Input: part model. Units: mm. Frame: model coordinates. Face numbers are marked on the shaded views. A direction names the side the tool comes from. Round coordinates to 2 decimals unless told otherwise and drop trailing zeros. Loops run counter-clockwise (first coordinate to the right, second up) from the corner with the lowest first, then second, coordinate; pieces in that order, holes last. Notation, with made-up numbers: (47.5, 75) - (74.5, 75) arc R7 cw to (74.5, 88) - close; hole circle Ø1 at (67, 34.5). An arc over 180 degrees is marked (long way). Use CSV: the item, a comma, the result in double quotes. Start each with the question number.
1. Pull-direction query (X, two-part tool) for the marked faces 3, 4 and 5; classes: +X half, -X half, draft (parallel to the pull), parting line (faces both ways), or undercut.
2. Cut plane C-C (x = -15). Return loops of the section in (y, z), and give its area (3 significant figures).
3. Cut plane A-A (z = 19). Return loops of the section in (x, y).
4. Material intervals for probe 1 along Y at (x, z) = (-14.4, 19); probe 2 along X at (y, z) = (-44.5, 1.75); probe 3 along Y at (x, z) = (-15.5, 21), sorted ascending. Write a range as from..to.
5. Pin query (flat end, axial travel): P1, Ø1.8, axis at y = -24.39, z = 9, coming from the -X side; P2, Ø0.8, axis at x = -15.5, z = 15.5, coming from the -Y side; P3, Ø6.5, axis at y = -38.43, z = 22, coming from the -X side; P4, Ø2.5, axis at y = -24.39, z = 19, coming from the +X side. Return the tip coordinate at first contact, or that it passes through.
6. Access query for the marked faces 1 and 2. Directions: +Z, -Z, +X, -X, +Y, -Y. A direction counts if a zero-diameter tool reaches every point of the face in a straight line with its end or side. Return the directions, or none.
7. Cut plane B-B (y = -38). Return loops of the section in (x, z), and give its area (3 significant figures).
8. Cut plane D-D (z = 2.5). Return loops of the section in (x, y), and give its area (3 significant figures).
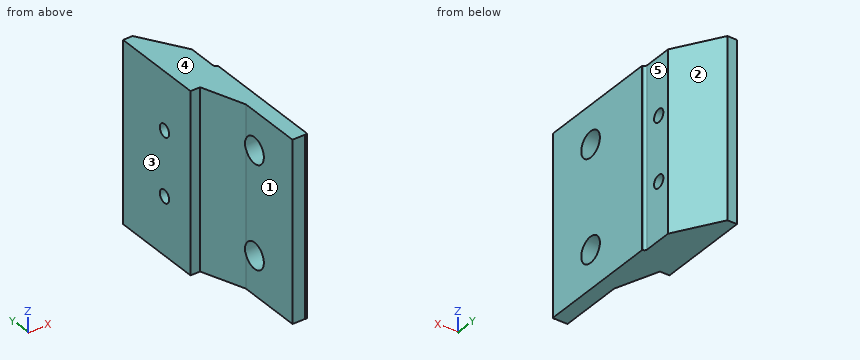
```python
from build123d import *

# Parameters (mm, degrees)
EXTRUDE_2_DEPTH          = 28
CUT_EXTRUDE_3_DEPTH      = 55.695457471
CUT_EXTRUDE_3_DEPTH_BACK = 55.695457471
SKETCH_2_R               = 1
SKETCH_2_R_2             = 2


with BuildPart() as part:
    # 草图1 → 凸台-拉伸2 (new body)
    with BuildSketch(Plane.XY):
        with BuildLine():
            Line((-15.852639514, -15.493363478), (-14.352639514, -15.493363478))
            Line((-14.352639514, -15.493363478), (-10.082641686, -22.391510936))
            Line((-10.082641686, -22.391510936), (-10.082641686, -26.891510936))
            ThreePointArc((-10.082641686, -26.891510936), (-9.999818758, -27.135229432), (-9.78564816, -27.27802053))
            ThreePointArc((-9.78564816, -27.27802053), (-9.692275449, -27.33339509), (-9.641586108, -27.429391944))
            Line((-9.641586108, -27.429391944), (-9.641586108, -46.429391944))
            ThreePointArc((-9.641586108, -46.429391944), (-9.760568765, -46.612247597), (-9.975948009, -46.577536736))
            Line((-9.975948009, -46.577536736), (-10.975948009, -46.577536736))
            Line((-10.975948009, -46.577536736), (-11.975948009, -46.577536736))
            Line((-11.975948009, -46.577536736), (-11.975948009, -36.577536736))
            Line((-11.975948009, -36.577536736), (-14.352639514, -29.993363478))
            Line((-14.352639514, -29.993363478), (-15.852639514, -29.993363478))
            Line((-15.852639514, -29.993363478), (-15.852639514, -15.493363478))
        make_face()
    extrude(amount=EXTRUDE_2_DEPTH)

    # 草图2 → 切除-拉伸3 (cut, two sides: drawn at the far end of the back side and taken through both)
    with BuildSketch(Plane(origin=(-10.082641686, 0, 0), x_dir=(0, 0, -1), z_dir=(1, 0, 0)).offset(-CUT_EXTRUDE_3_DEPTH_BACK)):
        with Locations(Location((-19, -24.391510936, 0), (0, 0, 90))):
            Circle(SKETCH_2_R)
        with Locations(Location((-22, -38.429391944, 0), (0, 0, 90))):
            Circle(SKETCH_2_R_2)
        with Locations(Location((-6, -38.429391944, 0), (0, 0, 90))):
            Circle(SKETCH_2_R_2)
        with Locations(Location((-9, -24.391510936, 0), (0, 0, 90))):
            Circle(SKETCH_2_R)
    extrude(amount=CUT_EXTRUDE_3_DEPTH + CUT_EXTRUDE_3_DEPTH_BACK, mode=Mode.SUBTRACT)


solid = part.part
```
Established:
1,face 3,"-X half"
1,face 4,"draft"
1,face 5,"+X half"
2,outline,"(-29.99, 0) - (-15.49, 0) - (-15.49, 28) - (-29.99, 28) - close; hole circle Ø2 at (-24.39, 9); hole circle Ø2 at (-24.39, 19)"
2,area,"400 mm2"
3,outline,"(-15.85, -29.99) - (-14.35, -29.99) - (-11.98, -36.58) - (-11.98, -46.58) - (-9.98, -46.58) arc R0.2 ccw to (-9.64, -46.43) - (-9.64, -27.43) arc R0.2 ccw to (-9.79, -27.28) arc R0.4 cw to (-10.08, -26.89) - (-10.08, -25.39) - (-15.85, -25.39) - close; (-15.85, -23.39) - (-10.08, -23.39) - (-10.08, -22.39) - (-14.35, -15.49) - (-15.85, -15.49) - close"
4,probe 1,"y = -29.99..-25.39, -23.39..-15.49"
4,probe 2,"x = -11.98..-9.64"
4,probe 3,"y = -29.99..-15.49"
5,P1,"passes through"
5,P2,"stops at y = -29.99"
5,P3,"stops at x = -12.48"
5,P4,"stops at x = -10.08"
6,face 1,"+Z, -Z, -X, -Y"
6,face 2,"+Z, -Z, +X, +Y"
7,outline,"(-11.98, 0) - (-9.64, 0) - (-9.64, 4.05) - (-11.98, 4.05) - close; (-11.98, 7.95) - (-9.64, 7.95) - (-9.64, 20.05) - (-11.98, 20.05) - close; (-11.98, 23.95) - (-9.64, 23.95) - (-9.64, 28) - (-11.98, 28) - close"
7,area,"47.1 mm2"
8,outline,"(-15.85, -29.99) - (-14.35, -29.99) - (-11.98, -36.58) - (-11.98, -46.58) - (-9.98, -46.58) arc R0.2 ccw to (-9.64, -46.43) - (-9.64, -27.43) arc R0.2 ccw to (-9.79, -27.28) arc R0.4 cw to (-10.08, -26.89) - (-10.08, -22.39) - (-14.35, -15.49) - (-15.85, -15.49) - close"
8,area,"117 mm2"
